Build history of the part. All positions in model axes, mm. Coordinates: 2 decimals unless noted, no trailing zeros. Order: outer loops, then holes, each group sorted by start corner. A loop starts at its lowest first (then second) coordinate and runs counter-clockwise, first axis right, second up. Notation, with made-up numbers: (-15, 12) - (15, 12) arc R6 cw to (15, 20) - close; hole circle Ø7 at (30, -16.5). An arc over 180 degrees is marked (long way). One line per item, written item: value.
from build123d import *

# Parameters (mm, degrees)
BOSS_EXTRUDE1_DEPTH = 350


with BuildPart() as part:
    # Sketch1 → Boss-Extrude1 (new body)
    with BuildSketch(Plane.XY):
        with BuildLine():
            Line((-21, 9.005025253), (-21, 7.456))
            ThreePointArc((-21, 7.456), (-19.36, 5.816), (-21, 4.176))
            Line((-21, 4.176), (-21, 0.494974747))
            Line((-21, 0.494974747), (-20.505025253, 0))
            Line((-20.505025253, 0), (20.505025253, 0))
            Line((20.505025253, 0), (21, 0.494974747))
            Line((21, 0.494974747), (21, 4.176))
            ThreePointArc((21, 4.176), (19.36, 5.816), (21, 7.456))
            Line((21, 7.456), (21, 9.005025253))
            Line((21, 9.005025253), (20.505025253, 9.5))
            Line((20.505025253, 9.5), (-20.505025253, 9.5))
            Line((-20.505025253, 9.5), (-21, 9.005025253))
        make_face()
    extrude(amount=BOSS_EXTRUDE1_DEPTH)

    # Sketch2 → Cut-Revolve1 (revolve, cut)
    with BuildSketch(Plane(origin=(11.5, 0, 0), x_dir=(0, 0, -1), z_dir=(1, 0, 0)), mode=Mode.PRIVATE) as cut_revolve1_sk:
        Polygon((-15, 9.5), (-11, 9.5), (-11, 5), (-12.75, 5), (-12.75, 0), (-15, 0), align=None)
    revolve(cut_revolve1_sk.sketch.rotate(Axis((11.5, 0, 15), (0, 1, 0)), 180), axis=Axis((11.5, 0, 15), (0, 1, 0)), mode=Mode.SUBTRACT)

    # Sketch3 → Cut-Revolve2 (revolve, cut)
    with BuildSketch(Plane(origin=(11.5, 0, 0), x_dir=(0, 0, -1), z_dir=(1, 0, 0)), mode=Mode.PRIVATE) as cut_revolve2_sk:
        Polygon((-335, 9.5), (-331, 9.5), (-331, 5), (-332.75, 5), (-332.75, 0), (-335, 0), align=None)
    revolve(cut_revolve2_sk.sketch.rotate(Axis((11.5, 0, 335), (0, 1, 0)), 180), axis=Axis((11.5, 0, 335), (0, 1, 0)), mode=Mode.SUBTRACT)

    # Sketch4 → Cut-Revolve3 (revolve, cut)
    with BuildSketch(Plane(origin=(-11.5, 0, 0), x_dir=(0, 0, -1), z_dir=(1, 0, 0)), mode=Mode.PRIVATE) as cut_revolve3_sk:
        Polygon((-335, 9.5), (-331, 9.5), (-331, 5), (-332.75, 5), (-332.75, 0), (-335, 0), align=None)
    revolve(cut_revolve3_sk.sketch.rotate(Axis((-11.5, 0, 335), (0, 1, 0)), 180), axis=Axis((-11.5, 0, 335), (0, 1, 0)), mode=Mode.SUBTRACT)

    # Sketch5 → Cut-Revolve4 (revolve, cut)
    with BuildSketch(Plane(origin=(11.5, 0, 0), x_dir=(0, 0, -1), z_dir=(1, 0, 0)), mode=Mode.PRIVATE) as cut_revolve4_sk:
        Polygon((-295, 9.5), (-291, 9.5), (-291, 5), (-292.75, 5), (-292.75, 0), (-295, 0), align=None)
    revolve(cut_revolve4_sk.sketch.rotate(Axis((11.5, 0, 295), (0, 1, 0)), 180), axis=Axis((11.5, 0, 295), (0, 1, 0)), mode=Mode.SUBTRACT)

    # Sketch6 → Cut-Revolve5 (revolve, cut)
    with BuildSketch(Plane(origin=(-11.5, 0, 0), x_dir=(0, 0, -1), z_dir=(1, 0, 0)), mode=Mode.PRIVATE) as cut_revolve5_sk:
        Polygon((-295, 9.5), (-291, 9.5), (-291, 5), (-292.75, 5), (-292.75, 0), (-295, 0), align=None)
    revolve(cut_revolve5_sk.sketch.rotate(Axis((-11.5, 0, 295), (0, 1, 0)), 180), axis=Axis((-11.5, 0, 295), (0, 1, 0)), mode=Mode.SUBTRACT)

    # Sketch7 → Cut-Revolve6 (revolve, cut)
    with BuildSketch(Plane(origin=(11.5, 0, 0), x_dir=(0, 0, -1), z_dir=(1, 0, 0)), mode=Mode.PRIVATE) as cut_revolve6_sk:
        Polygon((-255, 9.5), (-251, 9.5), (-251, 5), (-252.75, 5), (-252.75, 0), (-255, 0), align=None)
    revolve(cut_revolve6_sk.sketch.rotate(Axis((11.5, 0, 255), (0, 1, 0)), 180), axis=Axis((11.5, 0, 255), (0, 1, 0)), mode=Mode.SUBTRACT)

    # Sketch8 → Cut-Revolve7 (revolve, cut)
    with BuildSketch(Plane(origin=(-11.5, 0, 0), x_dir=(0, 0, -1), z_dir=(1, 0, 0)), mode=Mode.PRIVATE) as cut_revolve7_sk:
        Polygon((-255, 9.5), (-251, 9.5), (-251, 5), (-252.75, 5), (-252.75, 0), (-255, 0), align=None)
    revolve(cut_revolve7_sk.sketch.rotate(Axis((-11.5, 0, 255), (0, 1, 0)), 180), axis=Axis((-11.5, 0, 255), (0, 1, 0)), mode=Mode.SUBTRACT)

    # Sketch9 → Cut-Revolve8 (revolve, cut)
    with BuildSketch(Plane(origin=(11.5, 0, 0), x_dir=(0, 0, -1), z_dir=(1, 0, 0)), mode=Mode.PRIVATE) as cut_revolve8_sk:
        Polygon((-215, 9.5), (-211, 9.5), (-211, 5), (-212.75, 5), (-212.75, 0), (-215, 0), align=None)
    revolve(cut_revolve8_sk.sketch.rotate(Axis((11.5, 0, 215), (0, 1, 0)), 180), axis=Axis((11.5, 0, 215), (0, 1, 0)), mode=Mode.SUBTRACT)

    # Sketch10 → Cut-Revolve9 (revolve, cut)
    with BuildSketch(Plane(origin=(-11.5, 0, 0), x_dir=(0, 0, -1), z_dir=(1, 0, 0)), mode=Mode.PRIVATE) as cut_revolve9_sk:
        Polygon((-215, 9.5), (-211, 9.5), (-211, 5), (-212.75, 5), (-212.75, 0), (-215, 0), align=None)
    revolve(cut_revolve9_sk.sketch.rotate(Axis((-11.5, 0, 215), (0, 1, 0)), 180), axis=Axis((-11.5, 0, 215), (0, 1, 0)), mode=Mode.SUBTRACT)

    # Sketch11 → Cut-Revolve10 (revolve, cut)
    with BuildSketch(Plane(origin=(11.5, 0, 0), x_dir=(0, 0, -1), z_dir=(1, 0, 0)), mode=Mode.PRIVATE) as cut_revolve10_sk:
        Polygon((-175, 9.5), (-171, 9.5), (-171, 5), (-172.75, 5), (-172.75, 0), (-175, 0), align=None)
    revolve(cut_revolve10_sk.sketch.rotate(Axis((11.5, 0, 175), (0, 1, 0)), 180), axis=Axis((11.5, 0, 175), (0, 1, 0)), mode=Mode.SUBTRACT)

    # Sketch12 → Cut-Revolve11 (revolve, cut)
    with BuildSketch(Plane(origin=(-11.5, 0, 0), x_dir=(0, 0, -1), z_dir=(1, 0, 0)), mode=Mode.PRIVATE) as cut_revolve11_sk:
        Polygon((-175, 9.5), (-171, 9.5), (-171, 5), (-172.75, 5), (-172.75, 0), (-175, 0), align=None)
    revolve(cut_revolve11_sk.sketch.rotate(Axis((-11.5, 0, 175), (0, 1, 0)), 180), axis=Axis((-11.5, 0, 175), (0, 1, 0)), mode=Mode.SUBTRACT)

    # Sketch13 → Cut-Revolve12 (revolve, cut)
    with BuildSketch(Plane(origin=(11.5, 0, 0), x_dir=(0, 0, -1), z_dir=(1, 0, 0)), mode=Mode.PRIVATE) as cut_revolve12_sk:
        Polygon((-135, 9.5), (-131, 9.5), (-131, 5), (-132.75, 5), (-132.75, 0), (-135, 0), align=None)
    revolve(cut_revolve12_sk.sketch.rotate(Axis((11.5, 0, 135), (0, 1, 0)), 180), axis=Axis((11.5, 0, 135), (0, 1, 0)), mode=Mode.SUBTRACT)

    # Sketch14 → Cut-Revolve13 (revolve, cut)
    with BuildSketch(Plane(origin=(-11.5, 0, 0), x_dir=(0, 0, -1), z_dir=(1, 0, 0)), mode=Mode.PRIVATE) as cut_revolve13_sk:
        Polygon((-135, 9.5), (-131, 9.5), (-131, 5), (-132.75, 5), (-132.75, 0), (-135, 0), align=None)
    revolve(cut_revolve13_sk.sketch.rotate(Axis((-11.5, 0, 135), (0, 1, 0)), 180), axis=Axis((-11.5, 0, 135), (0, 1, 0)), mode=Mode.SUBTRACT)

    # Sketch15 → Cut-Revolve14 (revolve, cut)
    with BuildSketch(Plane(origin=(11.5, 0, 0), x_dir=(0, 0, -1), z_dir=(1, 0, 0)), mode=Mode.PRIVATE) as cut_revolve14_sk:
        Polygon((-95, 9.5), (-91, 9.5), (-91, 5), (-92.75, 5), (-92.75, 0), (-95, 0), align=None)
    revolve(cut_revolve14_sk.sketch.rotate(Axis((11.5, 0, 95), (0, 1, 0)), 180), axis=Axis((11.5, 0, 95), (0, 1, 0)), mode=Mode.SUBTRACT)

    # Sketch16 → Cut-Revolve15 (revolve, cut)
    with BuildSketch(Plane(origin=(-11.5, 0, 0), x_dir=(0, 0, -1), z_dir=(1, 0, 0)), mode=Mode.PRIVATE) as cut_revolve15_sk:
        Polygon((-95, 9.5), (-91, 9.5), (-91, 5), (-92.75, 5), (-92.75, 0), (-95, 0), align=None)
    revolve(cut_revolve15_sk.sketch.rotate(Axis((-11.5, 0, 95), (0, 1, 0)), 180), axis=Axis((-11.5, 0, 95), (0, 1, 0)), mode=Mode.SUBTRACT)

    # Sketch17 → Cut-Revolve16 (revolve, cut)
    with BuildSketch(Plane(origin=(11.5, 0, 0), x_dir=(0, 0, -1), z_dir=(1, 0, 0)), mode=Mode.PRIVATE) as cut_revolve16_sk:
        Polygon((-55, 9.5), (-51, 9.5), (-51, 5), (-52.75, 5), (-52.75, 0), (-55, 0), align=None)
    revolve(cut_revolve16_sk.sketch.rotate(Axis((11.5, 0, 55), (0, 1, 0)), 180), axis=Axis((11.5, 0, 55), (0, 1, 0)), mode=Mode.SUBTRACT)

    # Sketch18 → Cut-Revolve17 (revolve, cut)
    with BuildSketch(Plane(origin=(-11.5, 0, 0), x_dir=(0, 0, -1), z_dir=(1, 0, 0)), mode=Mode.PRIVATE) as cut_revolve17_sk:
        Polygon((-55, 9.5), (-51, 9.5), (-51, 5), (-52.75, 5), (-52.75, 0), (-55, 0), align=None)
    revolve(cut_revolve17_sk.sketch.rotate(Axis((-11.5, 0, 55), (0, 1, 0)), 180), axis=Axis((-11.5, 0, 55), (0, 1, 0)), mode=Mode.SUBTRACT)

    # Sketch19 → Cut-Revolve18 (revolve, cut)
    with BuildSketch(Plane(origin=(-11.5, 0, 0), x_dir=(0, 0, -1), z_dir=(1, 0, 0)), mode=Mode.PRIVATE) as cut_revolve18_sk:
        Polygon((-15, 9.5), (-11, 9.5), (-11, 5), (-12.75, 5), (-12.75, 0), (-15, 0), align=None)
    revolve(cut_revolve18_sk.sketch.rotate(Axis((-11.5, 0, 15), (0, 1, 0)), 180), axis=Axis((-11.5, 0, 15), (0, 1, 0)), mode=Mode.SUBTRACT)


solid = part.part
1. Flat gauge pin, fed straight in: P1, Ø4, axis at x = -11.5, z = 334, coming from the +Y side. Where does the tip first touch, or does it go through?
Values found:
P1: stops at y = 5
2. Band-saw the part on A-A, the plane z = 311.5. Give the cut face in (x, y), and give its area (3 significant figures).
Values found:
outline: (-21, 0.49) - (-20.51, 0) - (20.51, 0) - (21, 0.49) - (21, 4.18) arc R1.64 cw to (21, 7.46) - (21, 9.01) - (20.51, 9.5) - (-20.51, 9.5) - (-21, 9.01) - (-21, 7.46) arc R1.64 cw to (-21, 4.18) - close
area: 390 mm2
3. Probe line 1 along X through (y, z) = (8.2, 295); line 2 along X through (y, z) = (7.25, 138); line 3 along X through (y, z) = (6.5, 227.5). List the from-to ranges inside material, lowest first.
Values found:
line 1: x = -21 to -15.5, -7.5 to 7.5, 15.5 to 21
line 2: x = -20.2 to -14.15, -8.85 to 8.85, 14.15 to 20.2
line 3: x = -19.51 to 19.51
